```python
from build123d import *

# Parameters (mm, degrees)
SKETCH1_R           = 5
SKETCH1_R_2         = 1
BOSS_EXTRUDE1_DEPTH = 3


with BuildPart() as part:
    # Sketch1 → Boss-Extrude1 (new body)
    with BuildSketch(Plane(origin=(0, 0, 0), x_dir=(1, 0, 0), z_dir=(0, 1, 0))):
        with BuildLine():
            Line((-65.25, 63), (-68.25, 63))
            Line((-68.25, 63), (-68.25, 68))
            ThreePointArc((-68.25, 68), (-67.957106781, 68.707106781), (-67.25, 69))
            Line((-67.25, 69), (-63.058671293, 69))
            ThreePointArc((-63.058671293, 69), (-59.396555712, 68.305316194), (-56.243242609, 66.317781894))
            Line((-56.243242609, 66.317781894), (-19.079799162, 31.705545266))
            ThreePointArc((-19.079799162, 31.705545266), (-11.196516404, 26.736709515), (-2.04122745, 25))
            Line((-2.04122745, 25), (1.54122745, 25))
            ThreePointArc((1.54122745, 25), (10.696516404, 26.736709515), (18.579799162, 31.705545266))
            Line((18.579799162, 31.705545266), (55.743242609, 66.317781894))
            ThreePointArc((55.743242609, 66.317781894), (58.896555712, 68.305316194), (62.558671293, 69))
            Line((62.558671293, 69), (67.25, 69))
            ThreePointArc((67.25, 69), (67.957106781, 68.707106781), (68.25, 68))
            Line((68.25, 68), (68.25, 63))
            Line((68.25, 63), (65.25, 63))
            Line((65.25, 63), (65.25, 64))
            ThreePointArc((65.25, 64), (64.957106781, 64.707106781), (64.25, 65))
            Line((64.25, 65), (62.047564147, 65))
            ThreePointArc((62.047564147, 65), (61.343356803, 64.824421389), (60.804007789, 64.338789355))
            Line((60.804007789, 64.338789355), (29.524060686, 17.964360684))
            ThreePointArc((29.524060686, 17.964360684), (26.342381101, 11.293830715), (25.25, 3.984538097))
            Line((25.25, 3.984538097), (25.25, -3.984538097))
            ThreePointArc((25.25, -3.984538097), (26.342381101, -11.293830715), (29.524060686, -17.964360684))
            Line((29.524060686, -17.964360684), (60.804007789, -64.338789355))
            ThreePointArc((60.804007789, -64.338789355), (61.343356803, -64.824421389), (62.047564147, -65))
            Line((62.047564147, -65), (64.25, -65))
            ThreePointArc((64.25, -65), (64.957106781, -64.707106781), (65.25, -64))
            Line((65.25, -64), (65.25, -63))
            Line((65.25, -63), (68.25, -63))
            Line((68.25, -63), (68.25, -68))
            ThreePointArc((68.25, -68), (67.957106781, -68.707106781), (67.25, -69))
            Line((67.25, -69), (62.808671293, -69))
            ThreePointArc((62.808671293, -69), (59.146555712, -68.305316194), (55.993242609, -66.317781894))
            Line((55.993242609, -66.317781894), (18.829799162, -31.705545266))
            ThreePointArc((18.829799162, -31.705545266), (10.946516404, -26.736709515), (1.79122745, -25))
            Line((1.79122745, -25), (-1.79122745, -25))
            ThreePointArc((-1.79122745, -25), (-10.946516404, -26.736709515), (-18.829799162, -31.705545266))
            Line((-18.829799162, -31.705545266), (-55.993242609, -66.317781894))
            ThreePointArc((-55.993242609, -66.317781894), (-59.146555712, -68.305316194), (-62.808671293, -69))
            Line((-62.808671293, -69), (-67, -69))
            ThreePointArc((-67, -69), (-67.707106781, -68.707106781), (-68, -68))
            Line((-68, -68), (-68, -63))
            Line((-68, -63), (-65.25, -63))
            Line((-65.25, -63), (-65.25, -64))
            ThreePointArc((-65.25, -64), (-64.957106781, -64.707106781), (-64.25, -65))
            Line((-64.25, -65), (-62.047564147, -65))
            ThreePointArc((-62.047564147, -65), (-61.343356803, -64.824421389), (-60.804007789, -64.338789355))
            Line((-60.804007789, -64.338789355), (-29.524060686, -17.964360684))
            ThreePointArc((-29.524060686, -17.964360684), (-26.342381101, -11.293830715), (-25.25, -3.984538097))
            Line((-25.25, -3.984538097), (-25.25, 3.984538097))
            ThreePointArc((-25.25, 3.984538097), (-26.342381101, 11.293830715), (-29.524060686, 17.964360684))
            Line((-29.524060686, 17.964360684), (-60.804007789, 64.338789355))
            ThreePointArc((-60.804007789, 64.338789355), (-61.343356803, 64.824421389), (-62.047564147, 65))
            Line((-62.047564147, 65), (-64.25, 65))
            ThreePointArc((-64.25, 65), (-64.957106781, 64.707106781), (-65.25, 64))
            Line((-65.25, 64), (-65.25, 63))
        make_face()
        Circle(SKETCH1_R, mode=Mode.SUBTRACT)
        with Locations((0, 7.92)):
            Circle(SKETCH1_R_2, mode=Mode.SUBTRACT)
    extrude(amount=BOSS_EXTRUDE1_DEPTH)


solid = part.part
```
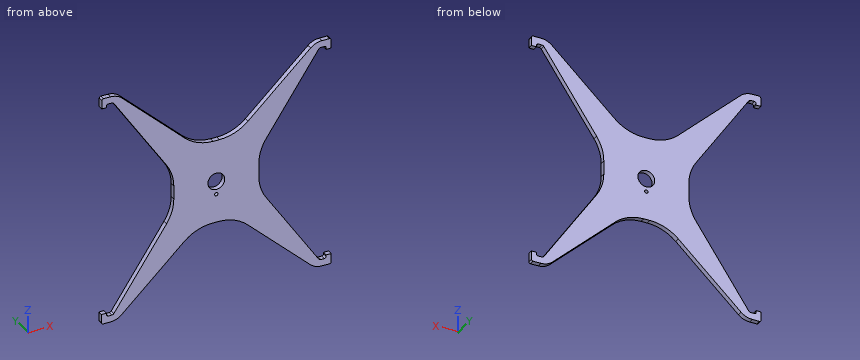
Here's how the part is built. I have some questions about the finished solid (model axes, mm). Give positions to 0.01 mm unless a question says otherwise; leave off trailing zeros. Loops run counter-clockwise (first coordinate to the right, second up) from the corner with the lowest first, then second, coordinate; pieces in that order, holes last. Notation, with made-up numbers: M -13,-30 L 18,-30 A20 cw 18,-26 Z; hole C 9.25,-17.75 d9. An arc over 180 degrees is marked long. Return JSON: item names as keys, results as strings.
Item 1: Imagine slicing it at C-C on y = 0.95. State how many separate pieces and enclosed holes the cut face has, then the cut area to 3 significant figures.
A:
{"separate pieces": "1", "enclosed holes": "2", "area": "5,300 mm^2"}
Item 2: Please list where these lines run through material, in increasing order: line 1 (Z direction, x = 0, y = 1.3); line 2 (X direction, y = 1.35, z = 0); line 3 (X direction, y = 2.25, z = -7.92).
A:
{"line 1": "z = -25 to -8.92, -6.92 to -5, 5 to 25", "line 2": "x = -25.25 to -5, 5 to 25.25", "line 3": "x = -25.56 to -1, 1 to 25.56"}
Item 3: Imagine slicing it at A-A on z = 0. List the corners of the cut face in (x, y) for me.
A:
{"outline": "M -25.25,0 L -5,0 L -5,3 L -25.25,3 Z; M 5,0 L 25.25,0 L 25.25,3 L 5,3 Z"}
Item 4: I'm going to push flat-ended pins straight in: pin 1 Ø1.5 at (x, z) = (-48, 41) entering from -Y; pin 2 Ø1 at (y, z) = (2, 44.5) entering from +X; pin 3 Ø1.1 at (y, z) = (1.5, 63.5) entering from -X; pin 4 Ø1 at (x, y) = (17.5, 0.5) entering from +Z. Where does each tip first touch, or does it pass through?
A:
{"pin 1": "passes through", "pin 2": "stops at x = 47.76", "pin 3": "stops at x = -68", "pin 4": "stops at z = 30.97"}
Item 5: Imagine slicing it at B-B on x = -52. List the corners of the cut face in (y, z) for me.
A:
{"outline": "M 0,-62.37 L 3,-62.37 L 3,-51.29 L 0,-51.29 Z; M 0,51.29 L 3,51.29 L 3,62.6 L 0,62.6 Z"}
